```python
from build123d import *

# Parameters (mm, degrees)
SKETCH2_R           = 8
SKETCH2_R_2         = 2.55
BOSS_EXTRUDE1_DEPTH = 10.6
BOSS_EXTRUDE2_START = 0.2
SKETCH3_R           = 8
SKETCH3_R_2         = 2.55
BOSS_EXTRUDE2_DEPTH = 0.2


with BuildPart() as part:
    # Sketch1 → Revolve1 (revolve)
    with BuildSketch(Plane(origin=(0, 0, 0), x_dir=(0, 0, -1), z_dir=(1, 0, 0)), mode=Mode.PRIVATE) as revolve1_sk:
        Polygon((-0.645132269, 8), (-11.045132269, 8), (-11.045132269, 9.8), (-8.845132269, 12), (-2.845132269, 12), (-0.645132269, 9.8), align=None)
    revolve(revolve1_sk.sketch.rotate(Axis((0, 0, 0), (0, 0, 1)), 90), axis=Axis((0, 0, 0), (0, 0, 1)))

    # Sketch2 → Boss-Extrude1 (add)
    with BuildSketch(Plane.XY.offset(11.045132269)):
        Circle(SKETCH2_R)
        Circle(SKETCH2_R_2, mode=Mode.SUBTRACT)
    extrude(amount=-BOSS_EXTRUDE1_DEPTH)

    # Sketch3 → Boss-Extrude2 (add)
    with BuildSketch(Plane.XY.offset(11.045132269).offset(BOSS_EXTRUDE2_START)):
        Circle(SKETCH3_R)
        Circle(SKETCH3_R_2, mode=Mode.SUBTRACT)
    extrude(amount=-BOSS_EXTRUDE2_DEPTH)


solid = part.part
```
The model under review builds one solid part; all positions refer to its coordinate system, in mm. A direction names the side the tool comes from. Round coordinates to 2 decimals unless told otherwise and drop trailing zeros. Loops run counter-clockwise (first coordinate to the right, second up) from the corner with the lowest first, then second, coordinate; pieces in that order, holes last. Notation, with made-up numbers: M -37.75,25.25 L -33.75,25.25 A18 ccw -33.75,49.25 Z; hole C 73.25,71.25 d6. An arc over 180 degrees is marked long. Answer as a JSON object with one key per item and string values.
(1) Take a section at C-C on z = 6.75. Give the boundary of the cut face in (x, y).
Resolved:
{"outline": "C 0,0 d24; hole C 0,0 d5.1"}
(2) Clearance check with flat-ended pins moving along their axes: P1, Ø4, axis at x = 3.5, z = 3.5, coming from the +Y side; P2, Ø4, axis at y = -4, z = 6, coming from the +X side; P3, Ø4, axis at x = 4.5, z = 8, coming from the -Y side; P4, Ø4, axis at x = 0, y = 0, coming from the +Z side. State where each tip first meets the part, or that it passes through.
Resolved:
{"P1": "y = 11.91", "P2": "x = 11.83", "P3": "y = -11.74", "P4": "through"}
(3) Tool access review of faces 1 (the flat face through (-8.03, 1.5, 11.045)), 2 (the flat face through (-2, 2, 0.445)), 3 (the flat face through (8.03, -1.5, 0.645)): name each direction out of +Z, -Z, +X, -X, +Y, -Y from which nothing blocks a thin tool from reaching the whole face with its end or side.
Resolved:
{"face 1": "+Z", "face 2": "-Z, +X, -X, +Y, -Y", "face 3": "-Z"}
(4) To check wall thickness, follow line 1 along Y through (x, z) = (0, 3.25); line 2 along Y through (x, z) = (-2, 2.5); line 3 along X through (y, z) = (-2.25, 8). State the ranges of each line that lie inside material, in increasing order.
Resolved:
{"line 1": "-12 to -2.55, 2.55 to 12", "line 2": "-11.48 to -1.58, 1.58 to 11.48", "line 3": "-11.79 to -1.2, 1.2 to 11.79"}
(5) Take a section at A-A on x = 0. Give the boundary of the cut face in (y, z), and give its area (3 significant figures).
Resolved:
{"outline": "M -12,2.85 L -9.8,0.65 L -8,0.65 L -8,0.45 L -2.55,0.45 L -2.55,11.25 L -8,11.25 L -8,11.05 L -9.8,11.05 L -12,8.85 Z; M 2.55,0.45 L 8,0.45 L 8,0.65 L 9.8,0.65 L 12,2.85 L 12,8.85 L 9.8,11.05 L 8,11.05 L 8,11.25 L 2.55,11.25 Z", "area": "191 mm²"}
